Autodesk Inventor part; units mm, degrees
ref_plane "YZ Plane" through (0, 0, 0) normal (1, 0, 0) x (0, 1, 0)
ref_plane "XZ Plane" through (0, 0, 0) normal (0, 1, 0) x (-1, 0, 0)
ref_plane "XY Plane" through (0, 0, 0) normal (0, 0, 1) x (1, 0, 0)
sketch "スケッチ1" plane through (0, 0, 0) normal (0, 0, 1) x (1, 0, 0)
  line L0 (-5.6, 0) -> (5.6, 0)
  line L1 (0, 0) -> (0, 6.25) construction
  line L2 (0, 6.25) -> (-4, 6.25)
  line L3 (-4, 6.25) -> (-4, 17)
  line L4 (-4, 17) -> (0, 17)
  line L5 (0, 6.25) -> (4, 6.25)
  line L6 (4, 6.25) -> (4, 17)
  line L7 (4, 17) -> (0, 17)
  dimension "d32" = 6.25
  dimension "d33" = 4
  dimension "d34" = 10.75
revolve "回転1" add sketch "スケッチ1" angle 180 mid plane about axis through (-10, 0, 0) along (1, 0, 0)
sketch "スケッチ5" plane through (-4, 0, -17) normal (-1, 0, 0) x (0, 0, 1)
  line L0 (17, 0) -> (17, 3) construction
  arc A0 (25.7409, 3) -> (8.2591, 3) centre (17, 0) ccw
  arc A1 (33.7332, 3) -> (0.2668, 3) centre (17, 0) ccw
  line L1 (0.2668, 3) -> (8.2668, 3)
  line L2 (33.7332, 3) -> (25.7332, 3.0224)
  circle A2 centre (17, 0) radius 9.2341
  point P0 (8.2591, 3)
  dimension "d35" = 3
  dimension "d49" = 8
  dimension "d50" = 8
extrude "押し出し2" cut sketch "スケッチ5" against normal through all contours A0 L1 A1 L2
sketch "スケッチ7" plane through (-4, 3.0224, 8.7332) normal (0, 1, 0.0028) x (1, 0, 0)
  line L0 (8, -8) -> (0, -8)
  line L1 (0, -8) -> (0, 0)
  point P0 (4, 8.7247)
  point P1 (4, -4)
  dimension "d51" = 4
  dimension "d52" = 4
hole "穴4" at (0, 3.0112, 12.7332) direction (0, -1, -0.0028) diameter 4.5 end through all
mirror "ミラー3" about plane through (0, 0, 0) normal (0, 0, 1) of "穴4"
properties part number "probe-cover-clump" material "ステンレス鋼"
Verification items for the finished model (mm, model axes). A direction names the side the tool comes from. Coordinates: 2 decimals unless noted, no trailing zeros. Loops run counter-clockwise (first coordinate to the right, second up) from the corner with the lowest first, then second, coordinate; pieces in that order, holes last. Notation, with made-up numbers: (-35, 69) -> (-21, 69) arc R18 cw to (-21, 91) -> close; hole circle Ø11 at (44, -5.75). An arc over 180 degrees is marked (long way). Answer in a Markdown table with one row per item. Add a question column.
1. Material ranges on probe 1 along Z at (x, y) = (-0.5, 2.75); probe 2 along Z at (x, y) = (-0.75, 5.5); probe 3 along Z at (x, y) = (-2, 2.5), recorded low to high. Write a range as [from, to].
2. Draft check along Z on faces 3 (the face through (-0.06, 6.25, 0.14)), 4 (the face through (-0.94, 0, 10.51)), 5 (the face through (0.056, 1.485, -16.935)), 6 (the face through (-0.1, 1.49, 10.48)). Enter one of: +Z half, -Z half, draft (parallel to the pull), parting line (faces both ways), or undercut.
3. Section check A-A, the plane y = 2.25. Give the number of separate pieces and of enclosed holes in the cut face, then the cut area to 3 significant figures.
4. Depth check by flat-ended pin: P1, Ø4, axis at x = -2, y = 6.5, coming from the -Z side; P2, Ø4, axis at x = 2, z = -6.5, coming from the +Y side; P3, Ø5, axis at y = 4.5, z = -13, coming from the -X side; P4, Ø1, axis at x = 1.5, z = -11, coming from the +Y side. Enter the tip coordinate at first touch or a pass-through.
5. Access from +Z, -Z, +X, -X, +Y, -Y to the whole of each face (thin tool, end or side, straight path). Record for faces 1 (the face through (-2, 3, -11)), 2 (the face through (-0.94, 0, -10.51)).
6. Section check C-C, the plane y = 8.25. Enter the section's corners in (x, z), then the cut area to 3 significant figures.
7. Section check B-B, the plane z = 0. Enter the section's corners in (x, y), then the cut area to 3 significant figures.
Derived:
| question | item | result |
|---|---|---|
| 1 | probe 1 | z = [-16.78, -14.93], [-10.54, -5.61], [5.61, 10.54], [14.93, 16.78] |
| 1 | probe 2 | z = [-7.43, -2.97], [2.97, 7.43] |
| 1 | probe 3 | z = [-16.82, -13.76], [-11.7, -5.73], [5.73, 11.7], [13.76, 16.82] |
| 2 | face 3 | undercut |
| 2 | face 4 | draft |
| 2 | face 5 | -Z half |
| 2 | face 6 | undercut |
| 3 | separate pieces | 2 |
| 3 | enclosed holes | 2 |
| 3 | area | 145 mm² |
| 4 | P1 | stops at z = -8.07 |
| 4 | P2 | stops at y = 8.07 |
| 4 | P3 | stops at x = -4 |
| 4 | P4 | stops at y = 3 |
| 5 | face 1 | -Z, +X, -X, +Y |
| 5 | face 2 | +Z, -Z, +X, -X, -Y |
| 6 | outline | (-4, -4.16) -> (4, -4.16) -> (4, 4.16) -> (-4, 4.16) -> close |
| 6 | area | 66.6 mm² |
| 7 | outline | (-4, 6.25) -> (4, 6.25) -> (4, 9.24) -> (-4, 9.24) -> close |
| 7 | area | 23.9 mm² |
